```python
from build123d import *

# Parameters (mm, degrees)
SKETCH1_W           = 1400
SKETCH1_H           = 600
BOSS_EXTRUDE1_DEPTH = 20
SKETCH2_W           = 20
SKETCH2_H           = 445
BOSS_EXTRUDE2_DEPTH = 720
SKETCH3_W           = 1200
SKETCH3_H           = 20
BOSS_EXTRUDE3_DEPTH = 450
SKETCH4_W           = 1200
SKETCH4_H           = 150
BOSS_EXTRUDE4_DEPTH = 20


with BuildPart() as part:
    # Sketch1 → Boss-Extrude1 (new body)
    with BuildSketch(Plane(origin=(0, 0, 0), x_dir=(1, 0, 0), z_dir=(0, 1, 0))):
        Rectangle(SKETCH1_W, SKETCH1_H)
    extrude(amount=-BOSS_EXTRUDE1_DEPTH)

    # Sketch2 → Boss-Extrude2 (add)
    with BuildSketch(Plane.XZ.offset(20)):
        with Locations((610, 0)):
            Rectangle(SKETCH2_W, SKETCH2_H)
        with Locations((-610, 0)):
            Rectangle(SKETCH2_W, SKETCH2_H)
    extrude(amount=BOSS_EXTRUDE2_DEPTH)

    # Sketch3 → Boss-Extrude3 (add)
    with BuildSketch(Plane.XZ.offset(20)):
        with Locations((0, -187.5)):
            Rectangle(SKETCH3_W, SKETCH3_H)
    extrude(amount=BOSS_EXTRUDE3_DEPTH)

    # Sketch4 → Boss-Extrude4 (add)
    with BuildSketch(Plane.XZ.offset(20)):
        with Locations((0, -102.5)):
            Rectangle(SKETCH4_W, SKETCH4_H)
        with Locations((0, 102.5)):
            Rectangle(SKETCH4_W, SKETCH4_H)
    extrude(amount=BOSS_EXTRUDE4_DEPTH)


solid = part.part
```
Build history of the part. All positions in model axes, mm. A direction names the side the tool comes from. Round coordinates to 2 decimals unless told otherwise and drop trailing zeros. Write each loop counter-clockwise with the first axis right and the second up, starting at its lowest first coordinate (ties: lowest second). Pieces come first, ordered by that corner, then holes. Notation, with made-up numbers: (60.25, 76) -> (117.25, 76) arc R30 ccw to (117.25, 109) -> close; hole circle Ø7 at (-12, -2). An arc over 180 degrees is marked (long way). Put each result on its own line as item: value.
Item 1: Flat gauge pins, fed straight in: P1, Ø22, axis at x = 103, y = -25.5, coming from the +Z side; P2, Ø1, axis at y = -152, z = 212, coming from the -X side; P3, Ø6, axis at x = 155.5, z = 178.5, coming from the -Y side; P4, Ø10, axis at x = 144.5, z = -187.5, coming from the -Y side. Where does each tip first touch, or does it go through?
Here are the results:
P1: stops at z = 300
P2: stops at x = -620
P3: stops at y = -40
P4: stops at y = -470
Item 2: Slice it at A-A, the plane y = -628.5. Give the cut face in (x, z), plus the area to 3 significant figures.
Here are the results:
outline: (-620, -222.5) -> (-600, -222.5) -> (-600, 222.5) -> (-620, 222.5) -> close; (600, -222.5) -> (620, -222.5) -> (620, 222.5) -> (600, 222.5) -> close
area: 17,800 mm^2
Item 3: Slice it at B-B, the plane x = -537. Give the cut face in (y, z), plus the area to 3 significant figures.
Here are the results:
outline: (-470, -197.5) -> (-20, -197.5) -> (-20, -300) -> (0, -300) -> (0, 300) -> (-20, 300) -> (-20, 177.5) -> (-40, 177.5) -> (-40, 27.5) -> (-20, 27.5) -> (-20, -27.5) -> (-40, -27.5) -> (-40, -177.5) -> (-470, -177.5) -> close
area: 27,000 mm^2
Item 4: Slice it at D-D, the plane y = -259.5. Give the cut face in (x, z).
Here are the results:
outline: (-620, -222.5) -> (-600, -222.5) -> (-600, -197.5) -> (600, -197.5) -> (600, -222.5) -> (620, -222.5) -> (620, 222.5) -> (600, 222.5) -> (600, -177.5) -> (-600, -177.5) -> (-600, 222.5) -> (-620, 222.5) -> close
Item 5: Wall check: probe 1 along X at (y, z) = (-124.5, -168.5); probe 2 along Y at (x, z) = (-364.5, -51); probe 3 along Y at (x, z) = (-355, -178.5). Give the ranges that are in metal, low to high. Write a range as from..to.
Here are the results:
probe 1: x = -620..-600, 600..620
probe 2: y = -40..0
probe 3: y = -470..0
Item 6: Slice it at C-C, the plane z = 113. Give the cut face in (x, y).
Here are the results:
outline: (-700, -20) -> (-620, -20) -> (-620, -740) -> (-600, -740) -> (-600, -40) -> (600, -40) -> (600, -740) -> (620, -740) -> (620, -20) -> (700, -20) -> (700, 0) -> (-700, 0) -> close
Item 7: Two-plate mould, pull along X, no slides. Class faces 1 (the face through (-600, -375, -3)), 2 (the face through (-10, 0, -4)), 3 (the face through (-620, -375, -3)): pulls with the +X half, pulls with the -X half, needs draft (parallel to the pull), parting line crosses it, or undercut.
Here are the results:
face 1: undercut
face 2: needs draft
face 3: pulls with the -X half
Item 8: Tool access for faces 4 (the face through (-8, -20, 0)), 5 (the face through (-8, -40, 104)), 6 (the face through (620, -375, -3)), 7 (the face through (-8, -242, -197.5)): list every direction of +Z, -Z, +X, -X, +Y, -Y with a clear straight run to the whole face (end or side of a thin tool).
Here are the results:
face 4: -Y
face 5: +Z, -Y
face 6: +Z, -Z, +X, -Y
face 7: -Z, -Y
